Build history of the part. All positions in model axes, mm. Give positions to 0.01 mm unless a question says otherwise; leave off trailing zeros. Write each loop counter-clockwise with the first axis right and the second up, starting at its lowest first coordinate (ties: lowest second). Pieces come first, ordered by that corner, then holes. Notation, with made-up numbers: (61, 34) -> (103, 34) arc R16 cw to (103, 45) -> close; hole circle Ø3 at (-9, -8). An arc over 180 degrees is marked (long way). One line per question, with ' | ' between items. Start each with the question number.
(1) Band-saw the part on B-B, the plane z = 0.85. Give the cut face in (x, y), and give its area (3 significant figures).
(2) Band-saw the part on A-A, the plane y = 11.5. Give the cut face in (x, z).
(3) Drill centre lines: probe 1 along Y at (x, z) = (1, 2.75); probe 2 along X at (y, z) = (25, 2.55). Where is each one in solid material? Low to high. Write a range as from..to.
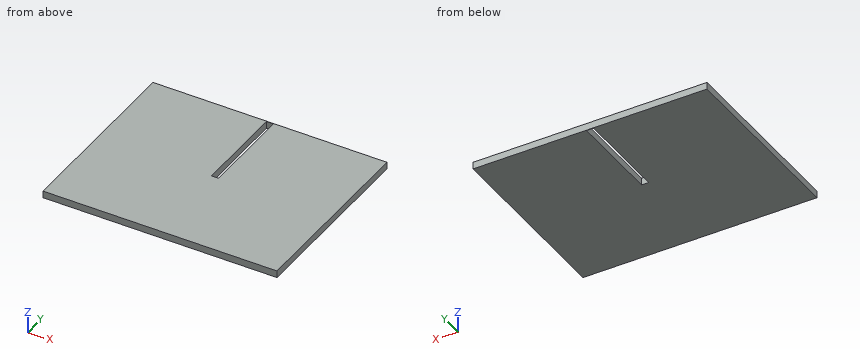
from build123d import *

# Parameters (mm, degrees)
SKETCH1_W               = 100
SKETCH1_H               = 80
BOSS_EXTRUDE1_DEPTH     = 3
CUT_EXTRUDE1_DEPTH      = 22
CUT_EXTRUDE1_DEPTH_BACK = 13
SKETCH2_W               = 3
SKETCH2_H               = 40


with BuildPart() as part:
    # Sketch1 → Boss-Extrude1 (new body)
    with BuildSketch(Plane.XY):
        Rectangle(SKETCH1_W, SKETCH1_H)
    extrude(amount=BOSS_EXTRUDE1_DEPTH)

    # Sketch2 → Cut-Extrude1 (cut, two sides: drawn at the far end of the back side and taken through both)
    with BuildSketch(Plane.XY.offset(3).offset(-CUT_EXTRUDE1_DEPTH_BACK)):
        with Locations((0.105052813, 19.789894374)):
            Rectangle(SKETCH2_W, SKETCH2_H)
    extrude(amount=CUT_EXTRUDE1_DEPTH + CUT_EXTRUDE1_DEPTH_BACK, mode=Mode.SUBTRACT)


solid = part.part
Results:
1) outline: (-50, -40) -> (50, -40) -> (50, 40) -> (-50, 40) -> close; hole (-1.39, -0.21) -> (1.61, -0.21) -> (1.61, 39.79) -> (-1.39, 39.79) -> close | area: 7,880 mm²
2) outline: (-50, 0) -> (-1.39, 0) -> (-1.39, 3) -> (-50, 3) -> close; (1.61, 0) -> (50, 0) -> (50, 3) -> (1.61, 3) -> close
3) probe 1: y = -40..-0.21, 39.79..40 | probe 2: x = -50..-1.39, 1.61..50
